Build history of the part. All positions in model axes, mm. Face numbers are marked on the shaded views. A direction names the side the tool comes from. Round coordinates to 2 decimals unless told otherwise and drop trailing zeros. Write each loop counter-clockwise with the first axis right and the second up, starting at its lowest first coordinate (ties: lowest second). Pieces come first, ordered by that corner, then holes. Notation, with made-up numbers: (-3, 70) -> (12, 70) arc R28 cw to (12, 103) -> close; hole circle Ø10 at (39, 11). An arc over 180 degrees is marked (long way). Answer in a Markdown table with one row per item. Add a question column.
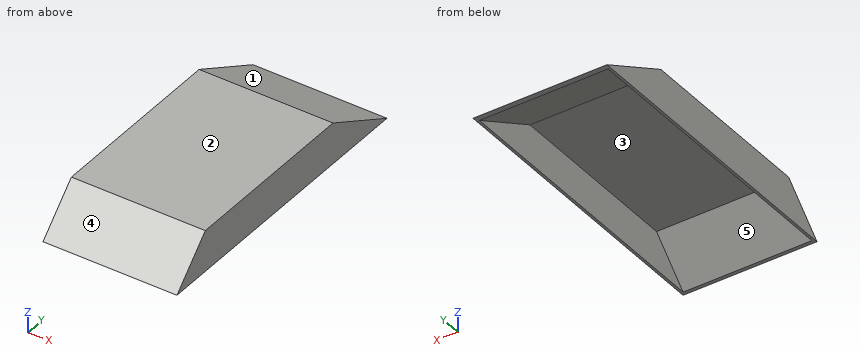
from build123d import *

# Parameters (mm, degrees)
F0_W     = 130
F0_H     = 296
F1_DEPTH = 20
F2_SIZE2 = 75.99999
F2_SIZE  = 39.99999
F3_SIZE2 = 39.99999
F3_SIZE  = 39.99999
F4_T     = 2.5


# Not quite as in the source:
# - a fillet or chamfer is up to 0.001 mm smaller than in the source, because OpenCascade refuses the exact size
# - a shell that OpenCascade refuses in one call is made with other operations: the cavity is built on its own and cut out


with BuildPart() as f1:
    # F0 (on Top) → F1 (new body, symmetric)
    with BuildSketch(Plane.XY):
        Rectangle(F0_W, F0_H)
    extrude(amount=F1_DEPTH, both=True)

    # F2 (size 40 and 76 in the source; OpenCascade refuses exactly that, so slightly less here)
    f2_edges = [f1.edges().sort_by_distance(p)[0] for p in [
        (0, 148, 20),
    ]]
    f2_side = f1.faces().sort_by_distance((0, 148, 0))[0]
    chamfer(f2_edges, length=F2_SIZE, length2=F2_SIZE2, reference=f2_side)

    # F3 (size 40 and 40 in the source; OpenCascade refuses exactly that, so slightly less here)
    f3_edges = [f1.edges().sort_by_distance(p)[0] for p in [
        (0, -148, 20),
    ]]
    chamfer(f3_edges, length=F3_SIZE, length2=F3_SIZE2)

    # F4: shell of thickness 2.5, made by hand


with BuildPart() as f4_core1:
    # F4_t2: copy of F1
    add(f1.part)

    # the walls: a layer under each face that stays
    f4_faces = [f4_core1.faces().sort_by_distance(p)[0] for p in [
        (-65, 0, 0),
        (0, -18, 20),
        (0, -128.000005, 5e-06),
        (0, 110.000005, 5e-06),
        (0, -148, -19.999995),
        (0, 148, -19.999995),
        (65, 0, 0),
    ]]
    thicken(f4_faces, amount=-F4_T, mode=Mode.SUBTRACT)


with BuildPart() as f1_1:
    add(f1.part)

    # what is left inside the walls is the cavity
    f4_cavity = [f4_core1.part.solids().sort_by_distance(p)[0] for p in [
        (0, -48.765554, -19.975),
    ]]
    add(f4_cavity, mode=Mode.SUBTRACT)


solid = f1_1.part
(1) Saw through at C-C (y = 21.5). List the corners of the cut face in (x, z).
(2) Drop flat-ended pins along their axis: P1, Ø8, axis at x = 48.5, y = -59, coming from the -Z side; P2, Ø8, axis at x = 12, y = 109.5, coming from the -Z side; P3, Ø12, axis at x = 35.5, z = -1, coming from the -Y side. Give the stop position or say it passes through.
(3) Mould opens along Y. For the marked faces 1, 2 and 3 say: pulls with the +Y half, pulls with the -Y half, needs draft (parallel to the pull), parting line crosses it, or undercut.
(4) Saw through at D-D (z = 13). List the corners of the cut face in (x, y).
(5) Which spindle directions (+Z, -Z, +X, -X, +Y, -Y) get a long thin tool onto all of the face, cutting with end or side? Do the marked faces 4 and 5. Say none if no direction does.
(6) Probe line 1 along X through (y, z) = (-105.5, 4); line 2 along Z through (x, y) = (38, -26.5); line 3 along Y through (x, z) = (28, 12). List the from-to ranges inside material, lowest first.
(7) Saw through at A-A (z = -13.5). List the corners of the cut face in (x, y), plus the area to 3 significant figures.
Answer sheet:
| question | item | result |
|---|---|---|
| 1 | outline | (-65, -20) -> (-62.5, -20) -> (-62.5, 17.5) -> (62.5, 17.5) -> (62.5, -20) -> (65, -20) -> (65, 20) -> (-65, 20) -> close |
| 2 | P1 | stops at z = 17.5 |
| 2 | P2 | stops at z = -4.67 |
| 2 | P3 | stops at y = -135 |
| 3 | face 1 | pulls with the +Y half |
| 3 | face 2 | needs draft |
| 3 | face 3 | undercut |
| 4 | outline | (-65, -115) -> (65, -115) -> (65, 85.3) -> (-65, 85.3) -> close; hole (-62.5, -111.46) -> (62.5, -111.46) -> (62.5, 79.93) -> (-62.5, 79.93) -> close |
| 5 | face 4 | +Z, +X, -X, -Y |
| 5 | face 5 | -Z |
| 6 | line 1 | x = -65 to -62.5, 62.5 to 65 |
| 6 | line 2 | z = 17.5 to 20 |
| 6 | line 3 | y = -116 to -112.46, 81.83 to 87.2 |
| 7 | outline | (-65, -141.5) -> (65, -141.5) -> (65, 135.65) -> (-65, 135.65) -> close; hole (-62.5, -137.96) -> (62.5, -137.96) -> (62.5, 130.28) -> (-62.5, 130.28) -> close |
| 7 | area | 2,500 mm² |
